Here's how the part is built. I have some questions about the finished solid (model axes, mm). Coordinates: 2 decimals unless noted, no trailing zeros. Order: outer loops, then holes, each group sorted by start corner. A loop starts at its lowest first (then second) coordinate and runs counter-clockwise, first axis right, second up. Notation, with made-up numbers: (37.25, 37.25) -> (43.25, 37.25) arc R38 cw to (43.25, 75.25) -> close; hole circle Ø11 at (32.25, -12.5). An arc over 180 degrees is marked (long way). One line per item, written item: value. Start each with the question number.
```python
from build123d import *

# Parameters (mm, degrees)
SKETCH1_W           = 12
SKETCH1_H           = 156
BOSS_EXTRUDE1_DEPTH = 3
CUT_EXTRUDE1_REACH  = 115.611
SKETCH2_R           = 2.1


with BuildPart() as part:
    # Sketch1 → Boss-Extrude1 (new body)
    with BuildSketch(Plane.XY):
        with Locations((76.55, 0)):
            Rectangle(SKETCH1_W, SKETCH1_H)
    extrude(amount=BOSS_EXTRUDE1_DEPTH)

    # Sketch2 → Cut-Extrude1 (cut, up to next)
    with BuildSketch(Plane(origin=(0, 0, 0), x_dir=(-1, 0, 0), z_dir=(0, 0, -1)), mode=Mode.PRIVATE) as cut_extrude1_sk1:
        with Locations((-76.55, -62)):
            Circle(SKETCH2_R)
    cut_extrude1_tool1 = extrude(cut_extrude1_sk1.sketch, amount=-CUT_EXTRUDE1_REACH, mode=Mode.PRIVATE) & part.part
    # Sketch2 → Cut-Extrude1 (cut, up to next)
    with BuildSketch(Plane(origin=(0, 0, 0), x_dir=(-1, 0, 0), z_dir=(0, 0, -1)), mode=Mode.PRIVATE) as cut_extrude1_sk2:
        with Locations((-76.55, 0)):
            Circle(SKETCH2_R)
    cut_extrude1_tool2 = extrude(cut_extrude1_sk2.sketch, amount=-CUT_EXTRUDE1_REACH, mode=Mode.PRIVATE) & part.part
    # Sketch2 → Cut-Extrude1 (cut, up to next)
    with BuildSketch(Plane(origin=(0, 0, 0), x_dir=(-1, 0, 0), z_dir=(0, 0, -1)), mode=Mode.PRIVATE) as cut_extrude1_sk3:
        with Locations((-76.55, 62)):
            Circle(SKETCH2_R)
    cut_extrude1_tool3 = extrude(cut_extrude1_sk3.sketch, amount=-CUT_EXTRUDE1_REACH, mode=Mode.PRIVATE) & part.part
    add(cut_extrude1_tool1.solids().sort_by_distance((76.55, -62, 0))[0], mode=Mode.SUBTRACT)
    add(cut_extrude1_tool2.solids().sort_by_distance((76.55, 0, 0))[0], mode=Mode.SUBTRACT)
    add(cut_extrude1_tool3.solids().sort_by_distance((76.55, 62, 0))[0], mode=Mode.SUBTRACT)


solid = part.part
```
Q1. Imagine slicing it at C-C (y = -62). Write out the boundary of the cut face in (x, z), plus the area to 3 significant figures.
Q2. Imagine slicing it at A-A (x = 76.55). Write out the boundary of the cut face in (y, z).
Q3. If we mould it in two halves opening along X, with no side actions, what happens to faces 1 (the face through (78.65, 0.09, 1.48)), 2 (the face through (79, 1, 0)), 3 (the face through (82.55, -1, 1))? For each: +X half, -X half, draft (parallel to the pull), parting line (faces both ways), or undercut.
Q4. For P1, Ø2.5, axis at x = 76.55, y = 0, coming from the +Z side, with a flat end and sliding along its axis, tell me the tip position at first contact or that it passes through.
Q5. Imagine slicing it at B-B (z = 1.25). Write out the boundary of the cut face in (x, y), plus the area to 3 significant figures.
Q6. I need wall thicknesses on line 1 (Y direction, x = 76.55, z = 1.05); line 2 (Y direction, x = 75.5, z = 2.25). Which ranges of each line are inside material? Lowest first, please.
Completed:
1. outline: (70.55, 0) -> (74.45, 0) -> (74.45, 3) -> (70.55, 3) -> close; (78.65, 0) -> (82.55, 0) -> (82.55, 3) -> (78.65, 3) -> close
1. area: 23.4 mm2
2. outline: (-78, 0) -> (-64.1, 0) -> (-64.1, 3) -> (-78, 3) -> close; (-59.9, 0) -> (-2.1, 0) -> (-2.1, 3) -> (-59.9, 3) -> close; (2.1, 0) -> (59.9, 0) -> (59.9, 3) -> (2.1, 3) -> close; (64.1, 0) -> (78, 0) -> (78, 3) -> (64.1, 3) -> close
3. face 1: undercut
3. face 2: draft
3. face 3: +X half
4. P1: passes through
5. outline: (70.55, -78) -> (82.55, -78) -> (82.55, 78) -> (70.55, 78) -> close; hole circle Ø4.2 at (76.55, -62); hole circle Ø4.2 at (76.55, 0); hole circle Ø4.2 at (76.55, 62)
5. area: 1,830 mm2
6. line 1: y = -78 to -64.1, -59.9 to -2.1, 2.1 to 59.9, 64.1 to 78
6. line 2: y = -78 to -63.82, -60.18 to -1.82, 1.82 to 60.18, 63.82 to 78
